Source: three-view drawing plus pictorial views. Frame: mm from the lowest corner of the part. Round coordinates to 2 decimals unless told otherwise and drop trailing zeros. Write each loop counter-clockwise with the first axis right and the second up, starting at its lowest first coordinate (ties: lowest second). Pieces come first, ordered by that corner, then holes.
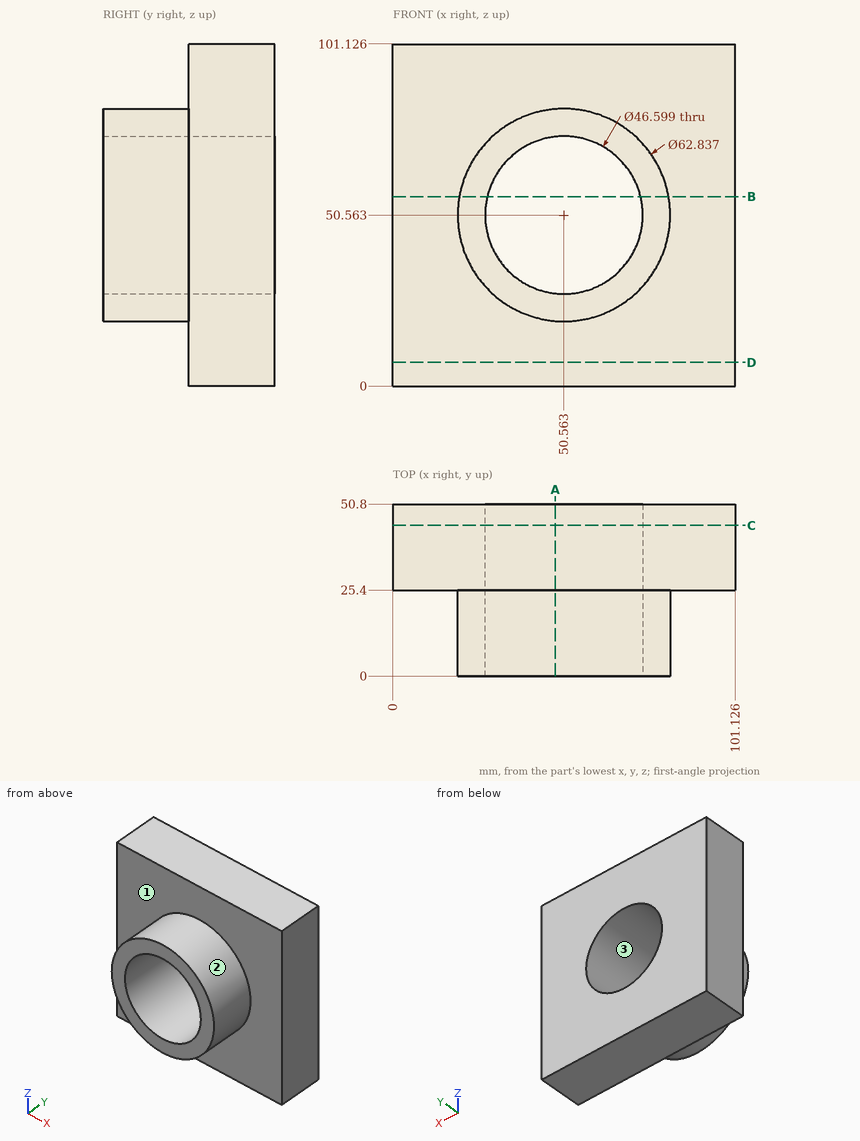
1) Section B-B on z = 56. Output: boundary loops of the cut face in (x, y), plus the area to 3 significant figures.
2) Line query: probe 1 along X at (y, z) = (47, 50.5); probe 2 along Y at (x, z) = (68, 80); probe 3 along X at (y, z) = (33, 55) (1 decimal). Output: solid intervals per line, ascending.
3) Section C-C on y = 44.5. Output: boundary loops of the cut face in (x, z).
4) Draft query along Z for the marked faces 1, 2 and 3. Return one class per face: pulls with the +Z half, pulls with the -Z half, needs draft (parallel to the pull), parting line crosses it, or undercut.
5) First-contact query: P1, Ø6, axis at y = 20.5, z = 53, coming from the +X side; P2, Ø4, axis at y = 15, z = 27, coming from the +X side; P3, Ø1, axis at x = 38.5, z = 15.5, coming from the -Y side. Flat tips, straight axial feed; report the tip coordinate or a pass-through.
6) Section A-A on x = 48. Output: boundary loops of the cut face in (y, z) (1 decimal), plus the area to 3 significant figures.
7) Section D-D on z = 7. Output: boundary loops of the cut face in (x, y), plus the area to 3 significant figures.
Filled in:
1. outline: (0, 25.4) - (19.62, 25.4) - (19.62, 0) - (27.91, 0) - (27.91, 50.8) - (0, 50.8) - close; (73.22, 0) - (81.51, 0) - (81.51, 25.4) - (101.13, 25.4) - (101.13, 50.8) - (73.22, 50.8) - close
1. area: 1,840 mm2
2. probe 1: x = 0 to 27.26, 73.86 to 101.13
2. probe 2: y = 25.4 to 50.8
2. probe 3: x = 0 to 27.7, 73.4 to 101.1
3. outline: (0, 0) - (101.13, 0) - (101.13, 101.13) - (0, 101.13) - close; hole circle Ø46.6 at (50.56, 50.56)
4. face 1: needs draft
4. face 2: parting line crosses it
4. face 3: undercut
5. P1: stops at x = 81.98
5. P2: stops at x = 73.41
5. P3: stops at y = 25.4
6. outline: (0, 19.2) - (25.4, 19.2) - (25.4, 0) - (50.8, 0) - (50.8, 27.4) - (0, 27.4) - close; (0, 73.7) - (50.8, 73.7) - (50.8, 101.1) - (25.4, 101.1) - (25.4, 81.9) - (0, 81.9) - close
6. area: 1,810 mm2
7. outline: (0, 25.4) - (101.13, 25.4) - (101.13, 50.8) - (0, 50.8) - close
7. area: 2,570 mm2
